```python
from build123d import *

# Parameters (mm, degrees)
SKETCH_1_W          = 50
SKETCH_1_H          = 50
SKETCH_1_R          = 21.05
EXTRUDE_1_DEPTH     = 15
SKETCH_2_W          = 50
SKETCH_2_H          = 30
SKETCH_2_R          = 1.6
EXTRUDE_2_DEPTH     = 15
FILLET_1_R          = 3
SKETCH_3_R          = 1.75
CUT_EXTRUDE_1_DEPTH = 63.24949799
SKETCH_4_R          = 1.6
CUT_EXTRUDE_2_DEPTH = 63.24949799
EXTRUDE_START       = 20
SKETCH_5_R          = 1.75
SKETCH_5_W          = 50
SKETCH_5_H          = 15
EXTRUDE_3_DEPTH     = 20
FILLET_2_R          = 2
FILLET_3_R          = 5
SKETCH_6_W          = 20
SKETCH_6_H          = 7
CUT_EXTRUDE_3_DEPTH = 64.639610307
CUT_EXTRUDE_4_DEPTH = 70.821200219
FILLET_4_R          = 1


with BuildPart() as part:
    # 草图1 → 凸台-拉伸1 (new body)
    with BuildSketch(Plane(origin=(0, 0, 0), x_dir=(1, 0, 0), z_dir=(0, 1, 0))):
        Rectangle(SKETCH_1_W, SKETCH_1_H)
        with Locations(Location((0, 0, 0), (0, 0, 270))):
            Circle(SKETCH_1_R, mode=Mode.SUBTRACT)
    extrude(amount=EXTRUDE_1_DEPTH)

    # 草图2 → 凸台-拉伸2 (add)
    with BuildSketch(Plane(origin=(0, 15, 0), x_dir=(1, 0, 0), z_dir=(0, 1, 0))):
        with Locations((0, -40)):
            Rectangle(SKETCH_2_W, SKETCH_2_H)
        with Locations(Location((-15, -47.5, 0), (0, 0, 270))):
            Circle(SKETCH_2_R, mode=Mode.SUBTRACT)
        with Locations(Location((15, -47.5, 0), (0, 0, 270))):
            Circle(SKETCH_2_R, mode=Mode.SUBTRACT)
    extrude(amount=-EXTRUDE_2_DEPTH)

    # 圆角1
    fillet_1_edges = [part.edges().sort_by_distance(p)[0] for p in [
        (25, 7.5, 55),
        (-25, 7.5, 55),
        (-25, 7.5, -25),
        (25, 7.5, -25),
    ]]
    fillet(fillet_1_edges, radius=FILLET_1_R)

    # 草图3 → 切除-拉伸1 (cut, through all)
    with BuildSketch(Plane(origin=(0, 15, 0), x_dir=(1, 0, 0), z_dir=(0, 1, 0))):
        with Locations(Location((-15, -30, 0), (0, 0, 270))):
            Circle(SKETCH_3_R)
        with Locations(Location((15, -30, 0), (0, 0, 270))):
            Circle(SKETCH_3_R)
    extrude(amount=-CUT_EXTRUDE_1_DEPTH, mode=Mode.SUBTRACT)

    # 草图4 → 切除-拉伸2 (cut, through all)
    # profile 1 of 6: a face of its own
    with BuildSketch(Plane(origin=(0, 15, 0), x_dir=(1, 0, 0), z_dir=(0, 1, 0))):
        with BuildLine():
            Line((25, -40), (-25, -40))
            Line((-25, -40), (-25, -52))
            ThreePointArc((-25, -52), (-24.121320344, -54.121320344), (-22, -55))
            Line((-22, -55), (22, -55))
            ThreePointArc((22, -55), (24.121320344, -54.121320344), (25, -52))
            Line((25, -52), (25, -40))
        make_face()
        with Locations((-15, -47.5)):
            Circle(SKETCH_4_R, mode=Mode.SUBTRACT)
        with Locations((15, -47.5)):
            Circle(SKETCH_4_R, mode=Mode.SUBTRACT)
    # profile 2 of 6: a face of its own
    with BuildSketch(Plane(origin=(0, 15, 0), x_dir=(1, 0, 0), z_dir=(0, 1, 0))):
        with BuildLine():
            Line((-25, 22), (-25, -12))
            Line((-25, -12), (-20.784609691, -12))
            ThreePointArc((-20.784609691, -12), (-6.211657082, 23.182219831), (24, 0))
            ThreePointArc((24, 0), (23.182219831, -6.211657082), (20.784609691, -12))
            Line((20.784609691, -12), (25, -12))
            Line((25, -12), (25, 22))
            ThreePointArc((25, 22), (24.121320344, 24.121320344), (22, 25))
            Line((22, 25), (-22, 25))
            ThreePointArc((-22, 25), (-24.121320344, 24.121320344), (-25, 22))
        make_face()
    # profile 3 of 6: a face of its own
    with BuildSketch(Plane(origin=(0, 15, 0), x_dir=(1, 0, 0), z_dir=(0, 1, 0))):
        with BuildLine():
            ThreePointArc((24, 0), (-6.211657082, 23.182219831), (-20.784609691, -12))
            Line((-20.784609691, -12), (-17.294580076, -12))
            ThreePointArc((-17.294580076, -12), (-6.286954326, 20.089218633), (21.05, 0))
            ThreePointArc((21.05, 0), (20.089218633, -6.286954326), (17.294580076, -12))
            Line((17.294580076, -12), (20.784609691, -12))
            ThreePointArc((20.784609691, -12), (23.182219831, -6.211657082), (24, 0))
        make_face()
    # profile 4 of 6: a face of its own
    with BuildSketch(Plane(origin=(0, 15, 0), x_dir=(1, 0, 0), z_dir=(0, 1, 0))):
        with BuildLine():
            Line((-17.294580076, -12), (-20.784609691, -12))
            ThreePointArc((-20.784609691, -12), (0, -24), (20.784609691, -12))
            Line((20.784609691, -12), (17.294580076, -12))
            ThreePointArc((17.294580076, -12), (0, -21.05), (-17.294580076, -12))
        make_face()
    # profile 5 of 6: a face of its own
    with BuildSketch(Plane(origin=(0, 15, 0), x_dir=(1, 0, 0), z_dir=(0, 1, 0))):
        with BuildLine():
            ThreePointArc((24, 0), (-6.211657082, 23.182219831), (-20.784609691, -12))
            Line((-20.784609691, -12), (-17.294580076, -12))
            ThreePointArc((-17.294580076, -12), (-6.286954326, 20.089218633), (21.05, 0))
            ThreePointArc((21.05, 0), (20.089218633, -6.286954326), (17.294580076, -12))
            Line((17.294580076, -12), (20.784609691, -12))
            ThreePointArc((20.784609691, -12), (23.182219831, -6.211657082), (24, 0))
        make_face()
    # profile 6 of 6: a face of its own
    with BuildSketch(Plane(origin=(0, 15, 0), x_dir=(1, 0, 0), z_dir=(0, 1, 0))):
        with BuildLine():
            Line((-17.294580076, -12), (-20.784609691, -12))
            ThreePointArc((-20.784609691, -12), (0, -24), (20.784609691, -12))
            Line((20.784609691, -12), (17.294580076, -12))
            ThreePointArc((17.294580076, -12), (0, -21.05), (-17.294580076, -12))
        make_face()
    extrude(amount=-CUT_EXTRUDE_2_DEPTH, mode=Mode.SUBTRACT)

    # 草图5 → 凸台-拉伸3 (add)
    # profile 1 of 2: a face of its own
    with BuildSketch(Plane(origin=(0, 15, 0), x_dir=(1, 0, 0), z_dir=(0, 1, 0)).offset(EXTRUDE_START)):
        with BuildLine():
            Line((-25, -12), (-25, -40))
            Line((-25, -40), (25, -40))
            Line((25, -40), (25, -12))
            Line((25, -12), (20.784609691, -12))
            ThreePointArc((20.784609691, -12), (0, -24), (-20.784609691, -12))
            Line((-20.784609691, -12), (-25, -12))
        make_face()
        with Locations(Location((-15, -30, 0), (0, 0, 270))):
            Circle(SKETCH_5_R, mode=Mode.SUBTRACT)
        with Locations(Location((15, -30, 0), (0, 0, 270))):
            Circle(SKETCH_5_R, mode=Mode.SUBTRACT)
    # profile 2 of 2: a face of its own
    with BuildSketch(Plane(origin=(0, 15, 0), x_dir=(1, 0, 0), z_dir=(0, 1, 0)).offset(EXTRUDE_START)):
        with Locations((0, -47.5)):
            Rectangle(SKETCH_5_W, SKETCH_5_H)
        with Locations(Location((15, -47.5, 0), (0, 0, 270))):
            Circle(SKETCH_5_R, mode=Mode.SUBTRACT)
        with Locations(Location((-15, -47.5, 0), (0, 0, 270))):
            Circle(SKETCH_5_R, mode=Mode.SUBTRACT)
    extrude(amount=-EXTRUDE_3_DEPTH)

    # 圆角2
    fillet_2_edges = [part.edges().sort_by_distance(p)[0] for p in [
        (20.784609691, 17.5, 12),
        (-20.784609691, 17.5, 12),
        (-25, 17.5, 12),
        (25, 17.5, 12),
    ]]
    fillet(fillet_2_edges, radius=FILLET_2_R)

    # 圆角3
    fillet_3_edges = [part.edges().sort_by_distance(p)[0] for p in [
        (-25, 25, 55),
        (25, 25, 55),
        (-25, 7.5, 40),
        (25, 7.5, 40),
    ]]
    fillet(fillet_3_edges, radius=FILLET_3_R)

    # 草图6 → 切除-拉伸3 (cut, through all)
    with BuildSketch(Plane.XZ.offset(-15)):
        with Locations((0, 47.5)):
            Rectangle(SKETCH_6_W, SKETCH_6_H)
    extrude(amount=-CUT_EXTRUDE_3_DEPTH, mode=Mode.SUBTRACT)

    # 草图7 → 切除-拉伸4 (cut, through all)
    with BuildSketch(Plane.XZ):
        with BuildLine():
            Line((0, 37), (0, 28))
            ThreePointArc((0, 28), (6.150195286, 27.316205775), (12, 25.298221281))
            Line((12, 25.298221281), (12, 37))
            Line((12, 37), (0, 37))
        make_face()
        with BuildLine():
            ThreePointArc((-12, 25.298221281), (-6.150195286, 27.316205775), (0, 28))
            Line((0, 28), (0, 37))
            Line((0, 37), (-12, 37))
            Line((-12, 37), (-12, 25.298221281))
        make_face()
    extrude(amount=-CUT_EXTRUDE_4_DEPTH, mode=Mode.SUBTRACT)

    # 圆角4
    fillet_4_edges = [part.edges().sort_by_distance(p)[0] for p in [
        (10, 35, 47.5),
        (10, 25, 51),
        (0, 35, 44),
        (10, 25, 44),
        (-10, 35, 47.5),
        (-10, 25, 44),
        (0, 35, 51),
        (-10, 25, 51),
        (10, 15, 47.5),
        (0, 15, 51),
        (-10, 15, 47.5),
        (0, 15, 44),
        (0, 0, 37),
        (-12, 17.5, 37),
        (12, 0, 31.149110641),
        (12, 17.5, 37),
        (0, 0, 28),
        (12, 17.5, 25.298221281),
        (-12, 35, 31.149110641),
        (-12, 17.5, 25.298221281),
        (0, 35, 37),
        (12, 35, 31.149110641),
        (0, 35, 28),
        (-12, 0, 31.149110641),
    ]]
    fillet(fillet_4_edges, radius=FILLET_4_R)


solid = part.part
```
Design review of the part built by this model. Coordinates are the model's own, in mm. A direction names the side the tool comes from. Give positions to 0.01 mm unless a question says otherwise; leave off trailing zeros. Write each loop counter-clockwise with the first axis right and the second up, starting at its lowest first coordinate (ties: lowest second). Pieces come first, ordered by that corner, then holes. Notation, with made-up numbers: (-15, 71) - (6, 71) arc R20 cw to (6, 92) - close; hole circle Ø3 at (63, -39.75). An arc over 180 degrees is marked (long way). Return JSON: item names as keys, results as strings. Group by question number.
(1) To check wall thickness, follow probe 1 along X at (y, z) = (29, 47.5); probe 2 along Z at (x, y) = (-2, 31); probe 3 along X at (y, z) = (26, 48.5). State the ranges of each line that lie inside material, in increasing order.
(2) Mouldability with a two-part tool opening along Z and no side actions: class faces 1 (the cylindrical face through (16.18, 17.74, 28.71)), 2 (the cylindrical face through (-11.546, 17.731, 25.995)), 3 (the flat face through (0, 25, 55)), 4 (the flat face through (-0.3, 15, 42.6)) as +Z half, -Z half, draft (parallel to the pull), parting line (faces both ways), or undercut.
(3) We need section A-A, the plane y = 13. Give the boundary of the cut face in (x, z).
(4) Machinability: for faces 5 (the cylindrical face through (23, 7, 39)), 6 (the flat face through (0, 25, 51)), 7 (the cylindrical face through (24.4, 17.74, 12.57)), 8 (the cylindrical face through (-20.94, 17.26, 12.25)), which of the approach directions +Z, -Z, +X, -X, +Y, -Y give a long, thin tool a straight path to every point of the face, cutting with its end or side? Answer none if there is none.
(5) Insertion check: pin 1 (4.5 mm diameter, centred on x = -15, z = 47.5, fed in from -Y); pin 2 (3 mm diameter, centred on x = 15, z = 47.5, fed in from +Y); pin 3 (1 mm diameter, centred on x = 14.5, y = 11.5, fed in from +Z); pin 4 (2 mm diameter, centred on x = -4.5, y = 16.5, fed in from -Z). Each pin has a flat end and moves straight along its axis. Give the tip position at first contact, or say it passes through.
(6) We need section D-D, the plane x = 15. Give the boundary of the cut face in (y, z) (3 decimals).
(7) We need section B-B, the plane z = 47.5. Give the boundary of the cut face in (x, y).
(8) We need section C-C, the plane z = 22.5. Give the boundary of the cut face in (x, y).
Reported:
{
 "1": {"probe 1": "x = -25 to -16.75, -13.25 to -10, 10 to 13.25, 16.75 to 25", "probe 2": "z = 23.92 to 27.93, 37 to 44, 51 to 55", "probe 3": "x = -25 to -16.44, -13.56 to -10, 10 to 13.56, 16.44 to 25"},
 "2": {"face 1": "undercut", "face 2": "undercut", "face 3": "+Z half", "face 4": "draft"},
 "3": {"outline": "(-25, 14) arc R2 ccw to (-23, 12) - (-21.91, 12) arc R2 ccw to (-20.22, 12.92) arc R24 cw to (20.22, 12.92) arc R2 ccw to (21.91, 12) - (23, 12) arc R2 ccw to (25, 14) - (25, 35) arc R5 ccw to (20, 40) - (-20, 40) arc R5 ccw to (-25, 35) - close; hole circle Ø3.5 at (-15, 30); hole (-12, 26.83) arc R1 ccw to (-10.62, 25.91) arc R28 cw to (10.62, 25.91) arc R1 ccw to (12, 26.83) - (12, 36) arc R1 ccw to (11, 37) - (-11, 37) arc R1 ccw to (-12, 36) - close; hole circle Ø3.5 at (15, 30)"},
 "4": {"face 5": "+Z, +X, -Y", "face 6": "+Y, -Y", "face 7": "-Z, +X, +Y, -Y", "face 8": "-Z, +Y, -Y"},
 "5": {"pin 1": "stops at y = 15", "pin 2": "passes through", "pin 3": "stops at z = 40", "pin 4": "stops at z = 23.36"},
 "6": {"outline": "(0, 18.735) - (35, 18.735) - (35, 28.25) - (0, 28.25) - close; (0, 31.75) - (35, 31.75) - (35, 45.75) - (15, 45.75) - (15, 40) - (0, 40) - close; (15, 49.25) - (35, 49.25) - (35, 55) - (15, 55) - close"},
 "7": {"outline": "(-25, 15) - (-16.75, 15) - (-16.75, 35) - (-25, 35) - close; (-13.25, 15) - (-11, 15) arc R1 ccw to (-10, 16) - (-10, 34) arc R1 ccw to (-11, 35) - (-13.25, 35) - close; (10, 16) arc R1 ccw to (11, 15) - (13.25, 15) - (13.25, 35) - (11, 35) arc R1 ccw to (10, 34) - close; (16.75, 15) - (25, 15) - (25, 35) - (16.75, 35) - close"},
 "8": {"outline": "(-25, 0) - (-8.35, 0) - (-8.35, 35) - (-25, 35) - close; (8.35, 0) - (25, 0) - (25, 35) - (8.35, 35) - close"}
}
